Model file for the job. Use its own axes, mm. Give positions to 0.01 mm unless a question says otherwise; leave off trailing zeros. Loops run counter-clockwise (first coordinate to the right, second up) from the corner with the lowest first, then second, coordinate; pieces in that order, holes last. Notation, with made-up numbers: M 47,-27 L 105,-27 A24 ccw 105,9 Z; hole C 40.25,-12.75 d5. An arc over 180 degrees is marked long. Answer in a Markdown table with one row per item.
Autodesk Inventor part; units mm, degrees
ref_plane "YZ Plane" through (0, 0, 0) normal (1, 0, 0) x (0, 1, 0)
ref_plane "XZ Plane" through (0, 0, 0) normal (0, 1, 0) x (-1, 0, 0)
ref_plane "XY Plane" through (0, 0, 0) normal (0, 0, 1) x (1, 0, 0)
sketch "Esboço1" plane through (0, 0, 0) normal (0, 1, 0) x (-1, 0, 0)
  line L0 (-1.4434, -2.5) -> (-2.8868, 0)
  line L1 (-2.8868, 0) -> (-1.4434, 2.5)
  line L2 (-1.4434, 2.5) -> (1.4434, 2.5)
  line L3 (1.4434, 2.5) -> (2.8868, 0)
  line L4 (2.8868, 0) -> (1.4434, -2.5)
  line L5 (1.4434, -2.5) -> (-1.4434, -2.5)
  circle A0 centre (0, 0) radius 1.5
  point P0 (0, -2.5)
extrude "Extrusão1" add sketch "Esboço1" along normal blind 30
chamfer "Chanfro1" distance 0.5 angle 45 2 edges at (1.5, 30, 0) (1.5, 0, 0)
thread "Rosca1"
properties part number "suporte" material "Latão, amarelo macio, soldado"
Q1. Mould opens along X. For faces 1 (the face through (-2.155, 14.79, 1.267)), 2 (the face through (1.5, 14.8, -0.07)), 3 (the face through (0, 15, 2.5)) say: released by +X, released by -X, zero draft, split by the parting line, or undercut.
Reported:
| item | result |
|---|---|
| face 1 | released by -X |
| face 2 | undercut |
| face 3 | zero draft |
Q2. Probe probe 1 along Z at (x, y) = (0, 17.25); probe 2 along X at (y, z) = (6.5, -0.55); probe 3 along Z at (x, y) = (-0.95, 19.75). List the from-to ranges inside material, lowest first.
Reported:
| item | result |
|---|---|
| probe 1 | -2.5 to -1.5, 1.5 to 2.5 |
| probe 2 | -2.57 to -1.4, 1.4 to 2.57 |
| probe 3 | -2.5 to -1.16, 1.16 to 2.5 |
Q3. Saw through at C-C (x = 2.3). Give the cut face in (y, z), and give its area (3 significant figures).
Reported:
| item | result |
|---|---|
| outline | M 0,-1.02 L 30,-1.02 L 30,1.02 L 0,1.02 Z |
| area | 61.0 mm² |
Q4. Saw through at A-A (x = 0). Give the cut face in (y, z), and give its area (3 significant figures).
Reported:
| item | result |
|---|---|
| outline | M 0,-2.5 L 30,-2.5 L 30,-2 L 29.5,-1.5 L 0.5,-1.5 L 0,-2 Z; M 0,2 L 0.5,1.5 L 29.5,1.5 L 30,2 L 30,2.5 L 0,2.5 Z |
| area | 59.5 mm² |
Q5. Drop flat-ended pins along their axis: pin 1 (1.5 mm diameter, centred on x = 2, y = 13.5, fed in from -Z); pin 2 (2 mm diameter, centred on y = 3.5, z = -2, fed in from +X); pin 3 (2.5 mm diameter, centred on x = 0, z = 0, fed in from +Y); pin 4 (1 mm diameter, centred on x = 2, y = 15, fed in from -Z). Give the stop position or say it passes through.
Reported:
| item | result |
|---|---|
| pin 1 | z = -2.5 |
| pin 2 | x = 2.31 |
| pin 3 | through |
| pin 4 | z = -2.4 |
Q6. Saw through at B-B (y = 7.75). Give the cut face in (x, z), and give its area (3 significant figures).
Reported:
| item | result |
|---|---|
| outline | M -2.89,0 L -1.44,-2.5 L 1.44,-2.5 L 2.89,0 L 1.44,2.5 L -1.44,2.5 Z; hole C 0,0 d3 |
| area | 14.6 mm² |
